Model file for the job. Use its own axes, mm. A direction names the side the tool comes from. Coordinates: 2 decimals unless noted, no trailing zeros. Loops run counter-clockwise (first coordinate to the right, second up) from the corner with the lowest first, then second, coordinate; pieces in that order, holes last. Notation, with made-up numbers: M -36,64.25 L -24,64.25 A29 cw -24,97.25 Z; hole C -39,89 d6. An arc over 180 degrees is marked long. Write item = value, one per line. Start each with the question number.
from build123d import *

# Parameters (mm, degrees)
SKETCH_1_R        = 68.5
SKETCH_1_R_2      = 65.5
EXTRUDE_1_DEPTH   = 2
SKETCH_1_R_3      = 55
SKETCH_1_R_4      = 52
EXTRUDE_1_2_DEPTH = 2
SKETCH_2_R        = 87.5
SKETCH_2_R_2      = 37.5
EXTRUDE_2_DEPTH   = 2
SKETCH_3_R        = 87.5
SKETCH_3_R_2      = 85.5
EXTRUDE_3_DEPTH   = 75
FILLET_1_R        = 1.5


with BuildPart() as part:
    # Sketch 1 → Extrude 1 (new body)
    with BuildSketch(Plane(origin=(0, 0, 0), x_dir=(1, 0, 0), z_dir=(0, 1, 0))):
        with Locations(Location((0, 0, 0), (0, 0, 270))):
            Circle(SKETCH_1_R)
        with Locations(Location((0, 0, 0), (0, 0, 270))):
            Circle(SKETCH_1_R_2, mode=Mode.SUBTRACT)
    extrude(amount=EXTRUDE_1_DEPTH)



with BuildPart() as body_2:
    # Sketch 1 → Extrude 1 2 (new body)
    with BuildSketch(Plane(origin=(0, 0, 0), x_dir=(1, 0, 0), z_dir=(0, 1, 0))):
        with Locations(Location((0, 0, 0), (0, 0, 270))):
            Circle(SKETCH_1_R_3)
        with Locations(Location((0, 0, 0), (0, 0, 270))):
            Circle(SKETCH_1_R_4, mode=Mode.SUBTRACT)
    extrude(amount=EXTRUDE_1_2_DEPTH)


with BuildPart() as part_1:
    add(part.part)

    add(body_2.part)  # Extrude 2 merges body 2
    # Sketch 2 → Extrude 2 (add)
    with BuildSketch(Plane.XZ):
        with Locations(Location((0, 0, 0), (0, 0, 270))):
            Circle(SKETCH_2_R)
        with Locations(Location((0, 0, 0), (0, 0, 270))):
            Circle(SKETCH_2_R_2, mode=Mode.SUBTRACT)
    extrude(amount=EXTRUDE_2_DEPTH)

    # Sketch 3 → Extrude 3 (add)
    with BuildSketch(Plane.XZ.offset(2)):
        with Locations(Location((0, 0, 0), (0, 0, 270))):
            Circle(SKETCH_3_R)
        with Locations(Location((0, 0, 0), (0, 0, 270))):
            Circle(SKETCH_3_R_2, mode=Mode.SUBTRACT)
    extrude(amount=EXTRUDE_3_DEPTH)

    # Fillet 1
    fillet_1_edges = [part_1.edges().sort_by_distance(p)[0] for p in [
        (0, 2, -68.5),
        (0, 2, -52),
        (0, 2, -55),
        (0, 2, -65.5),
    ]]
    fillet(fillet_1_edges, radius=FILLET_1_R - 0.0001)  # a hair under: the kernel refuses the full size


solid = part_1.part
Item 1: 3-axis set-ups, long thin cutter, end or side, ignore diameter. For faces 1 (the cylindrical face through (84.772, -38.975, 11.13)), 2 (the flat face through (54, 0, 15)), 3 (the flat face through (-84, -77, -19)): which of +Z, -Z, +X, -X, +Y, -Y reach the whole face in a straight line?
Item 2: Cut at A-A (y = -32.5). Give the cut face in (x, z), plus the area to 3 significant figures.
Item 3: Pin check, flat tips, straight feed: pin 1 Ø10 at (y, z) = (-40, -59.5) entering from +X; pin 2 Ø6 at (x, z) = (-29, 49.5) entering from +Y; pin 3 Ø1 at (x, y) = (-19, -30) entering from +Z. Stop position of each tip, or through.
Item 4: Cut at B-B (z = -72.5). Give the cut face in (x, y).
Item 5: Pull direction X, two halves, no side cores. Call faces 4 (the flat face through (-18, -2, -37)), 5 (the flat face through (15.7, 0, -34.4)), 6 (the flat face through (-45, 0, 52)), 7 (the cylindrical face through (86.755, -37.961, 11.391)): +X half, -X half, draft (parallel to the pull), parting line (faces both ways), or undercut.
Item 6: Probe L1, parallel to X at y = -48, z = 0; L2, parallel to X at y = -1.55, z = 0; L3, parallel to Z at x = 27, y = -70.5. List the from-to ranges inside material, lowest first.
Reported:
q1.face_1 = -Y
q1.face_2 = +Y
q1.face_3 = +Z, -Z, +X, -X, -Y
q2.outline = C 0,0 d175; hole C 0,0 d171
q2.area = 1,090 mm^2
q3.pin_1 = 68.45
q3.pin_2 = 1.72
q3.pin_3 = 85.52
q4.outline = M -48.99,-77 L -45.32,-77 L -45.32,-2 L 45.32,-2 L 45.32,-77 L 48.99,-77 L 48.99,0 L -48.99,0 Z
q5.face_4 = undercut
q5.face_5 = undercut
q5.face_6 = draft
q5.face_7 = parting line
q6.L1 = -87.5 to -85.5, 85.5 to 87.5
q6.L2 = -87.5 to -37.5, 37.5 to 87.5
q6.L3 = -83.23 to -81.12, 81.12 to 83.23
